Read the model definition and answer for the solid it produces. Units are mm, in the model's axes. A direction names the side the tool comes from. Round coordinates to 2 decimals unless told otherwise and drop trailing zeros. Order: outer loops, then holes, each group sorted by start corner. A loop starts at its lowest first (then second) coordinate and runs counter-clockwise, first axis right, second up.
from build123d import *

# Parameters (mm, degrees)
PAD_DEPTH       = 125
POCKET_DEPTH    = 125.001
SKETCH002_W     = 11.5
SKETCH002_H     = 24.578663
POCKET001_DEPTH = 125.001
SKETCH003_W     = 5
SKETCH003_H     = 32.052196
POCKET002_DEPTH = 107
SKETCH004_R     = 2
POCKET003_DEPTH = 5
SKETCH005_R     = 5
POCKET004_DEPTH = 52.001
SKETCH006_W     = 33.133884
SKETCH006_H     = 39.241348
POCKET005_DEPTH = 5
POCKET006_DEPTH = 55.001


with BuildPart() as part:
    # Sketch001 → Pad (new body)
    with BuildSketch(Plane.XZ.offset(62.5)):
        Polygon((-40, 0), (-15, 55), (15, 55), (40, 0), align=None)
    extrude(amount=PAD_DEPTH)

    # Sketch (on Face6 of Pad) → Pocket (cut, through all)
    with BuildSketch(Plane.XZ.offset(187.5)):
        Polygon((-12.478369, 34), (12.478369, 34), (25, 3), (-25, 3), align=None)
    extrude(amount=-POCKET_DEPTH, mode=Mode.SUBTRACT)

    # Sketch002 (on Face5 of Pocket) → Pocket001 (cut, through all)
    with BuildSketch(Plane.XZ.offset(187.5)):
        with Locations((0, 38.710668)):
            Rectangle(SKETCH002_W, SKETCH002_H)
    extrude(amount=-POCKET001_DEPTH, mode=Mode.SUBTRACT)

    # Sketch003 (on Face5 of Pocket001) → Pocket002 (cut)
    with BuildSketch(Plane.XZ.offset(187.5)):
        with Locations((0.018413, 60.238085)):
            Rectangle(SKETCH003_W, SKETCH003_H)
    extrude(amount=-POCKET002_DEPTH, mode=Mode.SUBTRACT)

    # Sketch004 (on Face2 of Pocket002) → Pocket003 (cut)
    with BuildSketch(Plane(origin=(0, -62.5, 0), x_dir=(1, 0, 0), z_dir=(0, 0, -1))):
        with Locations((0, 62.5)):
            Circle(SKETCH004_R)
    extrude(amount=-POCKET003_DEPTH, mode=Mode.SUBTRACT)

    # Sketch005 (on Face11 of Pocket003) → Pocket004 (cut, through all)
    with BuildSketch(Plane(origin=(0, -62.5, 3), x_dir=(-1, 0, 0), z_dir=(0, 0, 1))):
        with Locations((0, 62.5)):
            Circle(SKETCH005_R)
    extrude(amount=POCKET004_DEPTH, mode=Mode.SUBTRACT)

    # Sketch006 (on Face2 of Pocket004) → Pocket005 (cut)
    with BuildSketch(Plane(origin=(0, -62.5, 0), x_dir=(1, 0, 0), z_dir=(0, 0, -1))):
        with Locations((0.007028, 86.620669)):
            Rectangle(SKETCH006_W, SKETCH006_H)
        with Locations((-0.007028, 38.379331)):
            Rectangle(SKETCH006_W, SKETCH006_H)
    extrude(amount=-POCKET005_DEPTH, mode=Mode.SUBTRACT)

    # Sketch007 (on Face2 of Pocket005) → Pocket006 (cut, through all)
    with BuildSketch(Plane(origin=(0, -62.5, 0), x_dir=(1, 0, 0), z_dir=(0, 0, -1))):
        with BuildLine():
            ThreePointArc((57.666743, 99.777191), (0.524103, 115.241774), (-56.756832, 100.297573))
            Line((-66.493973, 135.547501), (-56.756832, 100.297573))
            Line((80.722458, 130.041382), (-66.493973, 135.547501))
            Line((65.916746, 95.009059), (80.722458, 130.041382))
            Line((57.666743, 99.777191), (65.916746, 95.009059))
        make_face()
        with BuildLine():
            ThreePointArc((-48.384384, 71.931989), (1.820118, 56.580716), (51.310891, 74.096909))
            Line((51.310891, 74.096909), (53.523094, 75.808954))
            Line((53.523094, 75.808954), (72.60817, -29.346481))
            Line((72.60817, -29.346481), (-27.661308, -61.224059))
            Line((-27.661308, -61.224059), (-105.616463, 40.204582))
            Line((-105.616463, 40.204582), (-48.384384, 71.931989))
        make_face()
    extrude(amount=-POCKET006_DEPTH, mode=Mode.SUBTRACT)


solid = part.part
Q1. For a pull along Y with two mould halves and no side action, classify faces 1 (the face through (0, -120.5, 1)), 2 (the face through (0, -168.741, 1)), 3 (the face through (9, -149, 34)) as released by +Y, released by -Y, zero draft, split by the parting line, or undercut.
Outcome:
face 1: released by +Y
face 2: undercut
face 3: zero draft
Q2. A cutting plane is placed at B-B, the plane y = -136. Give the vertices of the cut face in (x, z), plus the area to 3 significant figures.
Outcome:
outline: (-40, 0) - (-16.56, 0) - (-16.56, 3) - (-25, 3) - (-12.48, 34) - (-5.75, 34) - (-5.75, 51) - (-2.48, 51) - (-2.48, 55) - (-15, 55) - close; (2.52, 51) - (5.75, 51) - (5.75, 34) - (12.48, 34) - (25, 3) - (16.57, 3) - (16.57, 0) - (40, 0) - (15, 55) - (2.52, 55) - close
area: 1,550 mm2
Q3. Flat-ended cylindrical pins translate along their axes: pin 1 (2 mm diameter, centred on x = -8.5, y = -152.5, fed in from -Z); pin 2 (1.2 mm diameter, centred on y = -164.5, z = 52.5, fed in from +X); pin 3 (1.5 mm diameter, centred on y = -141, z = 1.5, fed in from -X); pin 4 (3 mm diameter, centred on x = 20.5, z = 8.5, fed in from -Y). Find the tip coordinate at first contact, or state that the pin passes through.
Outcome:
pin 1: stops at z = 34
pin 2: stops at x = 16.41
pin 3: stops at x = -39.66
pin 4: passes through
Q4. Straight lines are drawn through the part: probe 1 along Z at (x, y) = (6.5, -127); probe 2 along Z at (x, y) = (23.5, -147); probe 3 along Z at (x, y) = (-3, -159.5). For each, find the intervals that lie inside material, in ascending order.
Outcome:
probe 1: z = 0 to 3, 34 to 55
probe 2: z = 0 to 3, 6.71 to 36.3
probe 3: z = 51 to 55
Q5. For faces 4 (the face through (-5.75, -149, 42)), 5 (the face through (16.574, -149, 1)), 6 (the face through (-17, -149, 0)), 7 (the face through (-5, -125, 53)), 8 (the face through (1.075, -126.686, 1.479)), determine the directions among +Z, -Z, +X, -X, +Y, -Y from which every point of the face is accessible in a straight line to the end or side of a thin tool.
Outcome:
face 4: +Y, -Y
face 5: -Z
face 6: -Z, +X, -X, +Y, -Y
face 7: +Z
face 8: +Z, -Z
Q6. A cutting plane is placed at D-D, the plane y = -125. Give the vertices of the cut face in (x, z), plus the area to 3 significant figures.
Outcome:
outline: (-30.99, 0) - (-2, 0) - (-2, 3) - (-25, 3) - (-12.48, 34) - (-5.75, 34) - (-5.75, 51) - (-5, 51) - (-5, 55) - (-15, 55) - (-30.99, 19.82) - close; (2, 0) - (30.99, 0) - (30.99, 19.82) - (15, 55) - (5, 55) - (5, 51) - (5.75, 51) - (5.75, 34) - (12.48, 34) - (25, 3) - (2, 3) - close
area: 1,440 mm2
Q7. A cutting plane is placed at C-C, the plane z = 37. Give the vertices of the cut face in (x, y).
Outcome:
outline: (-23.18, -175.39) arc R115.24 ccw to (-5.75, -177.6) - (-5.75, -119.26) arc R83.84 ccw to (-23.18, -122.33) - close; (5.75, -177.6) arc R115.24 ccw to (23.18, -175.39) - (23.18, -122.33) arc R83.84 ccw to (5.75, -119.26) - close
Q8. A cutting plane is placed at A-A, the plane x = 0. Give the vertices of the cut face in (y, z).
Outcome:
outline: (-177.74, 0) - (-168.74, 0) - (-168.74, 3) - (-177.74, 3) - close; (-129.5, 0) - (-127, 0) - (-127, 3) - (-129.5, 3) - close; (-123, 0) - (-120.5, 0) - (-120.5, 3) - (-123, 3) - close
